Can you work these out from the model? Positions are in its coordinate system, mm. A direction names the side the tool comes from. Give positions to 0.01 mm unless a question says otherwise; leave off trailing zeros. Order: outer loops, then holes, each group sorted by start corner. A loop starts at its lowest first (then second) coordinate and runs counter-clockwise, first axis right, second up.
```python
from build123d import *

# Parameters (mm, degrees)
F0_R     = 3
F1_DEPTH = 30
F0_R_2   = 1.75
F2_DEPTH = 26


with BuildPart() as f1:
    # F0 (on Top) → F1 (new body)
    with BuildSketch(Plane.XY):
        with BuildLine():
            ThreePointArc((-60, -64), (-57.1715728753, -62.8284271247), (-56, -60))
            ThreePointArc((-56, -60), (-57.1715728753, -57.1715728753), (-60, -56))
            ThreePointArc((-60, -56), (-62.8284271247, -57.1715728753), (-64, -60))
            ThreePointArc((-64, -60), (-62.8284271247, -62.8284271247), (-60, -64))
        make_face()
        with Locations((-60, -60)):
            Circle(F0_R, mode=Mode.SUBTRACT)
        with BuildLine():
            ThreePointArc((-64, -60), (-62.8284271247, -57.1715728753), (-60, -56))
            Line((-60, -56), (-64, -56))
            Line((-64, -56), (-64, -60))
        make_face()
        with BuildLine():
            Line((-61, -64), (-60, -64))
            ThreePointArc((-60, -64), (-62.8284271247, -62.8284271247), (-64, -60))
            Line((-64, -60), (-64, -61))
            Line((-64, -61), (-67, -61))
            Line((-67, -61), (-67, -56))
            Line((-67, -56), (-69, -56))
            Line((-69, -56), (-69, -64))
            ThreePointArc((-69, -64), (-67.5355339059, -67.5355339059), (-64, -69))
            Line((-64, -69), (-63.9991187476, -69))
            Line((-63.9991187476, -69), (-56, -69))
            Line((-56, -69), (-56, -67))
            Line((-56, -67), (-61, -67))
            Line((-61, -67), (-61, -64))
        make_face()
        with BuildLine():
            Line((-56, -64), (-56, -60))
            ThreePointArc((-56, -60), (-57.1715728753, -62.8284271247), (-60, -64))
            Line((-60, -64), (-56, -64))
        make_face()
    extrude(amount=F1_DEPTH)

    # F0 (on Top) → F2 (join)
    with BuildSketch(Plane.XY):
        with Locations((-60, -60)):
            Circle(F0_R)
        with Locations((-60, -60)):
            Circle(F0_R_2, mode=Mode.SUBTRACT)
    extrude(amount=F2_DEPTH)


solid = f1.part
```
1) I'm going to push flat-ended pins straight in: pin 1 Ø1.5 at (x, z) = (-65, 10.5) entering from +Y; pin 2 Ø3 at (x, y) = (-60.5, -59.5) entering from +Z; pin 3 Ø2 at (y, z) = (-66.5, 23.5) entering from -X. Where does each tip first touch, or does it pass through?
2) Suppose I cut it at A-A (z = 17.75). Please give me the cut outline in (x, y).
3) Suppose I cut it at B-B (x = -60.5). Please give me the cut outline in (y, z), and give its area (3 significant figures).
4) Suppose I cut it at C-C (y = -66). Please give me the cut outline in (x, z).
5) We'd pull the mould along Y, two halves only. Please class faces 1 (the face through (-59, -64, 15)), 2 (the face through (-63, -64, 30)), 3 (the face through (-57.141, -57.203, 14.79)): +Y half, -Y half, draft (parallel to the pull), parting line (faces both ways), or undercut.
6) Which directions (+Z, -Z, +X, -X, +Y, -Y) give clear straight access to the entire face, cutting with the end or side of a thin tool? Please do faces 4 (the face through (-63, -62, 0)), 5 (the face through (-58, -67, 15)), 6 (the face through (-67, -59, 15)), 7 (the face through (-68, -67, 15)), 8 (the face through (-60, -62, 26)).
7) If I drill on line 1 (Y direction, x = -60, z = 11.25); line 2 (X direction, y = -60.25, z = 3); line 3 (Y direction, x = -57.5, z = 23.5), over which ranges is the centre line in solid material (lowest first)?
Results:
1. pin 1: stops at y = -61
1. pin 2: stops at z = 26
1. pin 3: stops at x = -68.77
2. outline: (-69, -64) arc R5 ccw to (-64, -69) - (-56, -69) - (-56, -67) - (-61, -67) - (-61, -64) - (-56, -64) - (-56, -60) arc R4 ccw to (-60, -56) - (-64, -56) - (-64, -61) - (-67, -61) - (-67, -56) - (-69, -56) - close; hole circle Ø3.5 at (-60, -60)
3. outline: (-69, 0) - (-67, 0) - (-67, 30) - (-69, 30) - close; (-64, 0) - (-61.68, 0) - (-61.68, 26) - (-62.96, 26) - (-62.96, 30) - (-64, 30) - close; (-58.32, 0) - (-56, 0) - (-56, 30) - (-57.04, 30) - (-57.04, 26) - (-58.32, 26) - close
3. area: 189 mm2
4. outline: (-68.58, 0) - (-61, 0) - (-61, 30) - (-68.58, 30) - close
5. face 1: undercut
5. face 2: draft
5. face 3: +Y half
6. face 4: -Z, +X, -X, +Y, -Y
6. face 5: +Z, -Z, +X
6. face 6: +Z, -Z, +Y
6. face 7: +Z, -Z, -X, -Y
6. face 8: +Z
7. line 1: y = -69 to -67, -64 to -61.75, -58.25 to -56
7. line 2: x = -69 to -67, -64 to -61.73, -58.27 to -56
7. line 3: y = -69 to -67, -64 to -56.88
